```python
from build123d import *

# Parameters (mm, degrees)
SKETCH_1_W          = 10
SKETCH_1_H          = 20
SKETCH_1_R          = 1.65
EXTRUDE_1_DEPTH     = 27
FILLET_1_R          = 3
SKETCH_2_R          = 1.6
CUT_EXTRUDE_1_DEPTH = 36.057096286


with BuildPart() as part:
    # 草图1 → 凸台-拉伸1 (new body)
    with BuildSketch(Plane.XY):
        with Locations((5, -10)):
            Rectangle(SKETCH_1_W, SKETCH_1_H)
        with Locations((5, -5)):
            Circle(SKETCH_1_R, mode=Mode.SUBTRACT)
        with Locations((5, -15)):
            Circle(SKETCH_1_R, mode=Mode.SUBTRACT)
    extrude(amount=EXTRUDE_1_DEPTH)

    # 圆角1
    fillet_1_edges = [part.edges().sort_by_distance(p)[0] for p in [
        (0, 0, 13.5),
        (10, 0, 13.5),
        (10, -20, 13.5),
        (0, -20, 13.5),
    ]]
    fillet(fillet_1_edges, radius=FILLET_1_R)

    # 草图2 → 切除-拉伸1 (cut, through all)
    with BuildSketch(Plane(origin=(10, 0, 0), x_dir=(0, 0, -1), z_dir=(1, 0, 0))):
        with Locations(Location((-21, -10, 0), (0, 0, 90))):
            Circle(SKETCH_2_R)
        with Locations(Location((-6, -10, 0), (0, 0, 90))):
            Circle(SKETCH_2_R)
    extrude(amount=-CUT_EXTRUDE_1_DEPTH, mode=Mode.SUBTRACT)


solid = part.part
```
For this review, take the finished solid that the model builds, in its own axes (mm). Coordinates: 2 decimals unless noted, no trailing zeros. Loops run counter-clockwise (first coordinate to the right, second up) from the corner with the lowest first, then second, coordinate; pieces in that order, holes last.
1. Mouldability with a two-part tool opening along Y and no side actions: class faces 1 (the flat face through (0, -10, 13)), 2 (the flat face through (5, 0, 13)), 3 (the cylindrical face through (3.35, -4.93, 13.31)) as +Y half, -Y half, draft (parallel to the pull), parting line (faces both ways), or undercut.
2. Add section B-B, the plane z = 21. Give the boundary of the cut face in (x, y).
3. Insertion check: P1, Ø1, axis at x = 2, z = 12.5, coming from the -Y side; P2, Ø4, axis at x = 5, y = -15, coming from the +Z side. Each pin has a flat end and moves straight along its axis. Give the tip position at first contact, or say it passes through.
4. For line 1 (Y direction, x = 5, z = 19.25); line 2 (Y direction, x = 6.5, z = 18.5); line 3 (Y direction, x = 5, z = 7), list the stretches that pass through material, from the lowest coordinate up.
5. Add section A-A, the plane x = 5. Give the boundary of the cut face in (y, z), then the cut area to 3 significant figures.
6. Add section D-D, the plane y = -10. Give the boundary of the cut face in (x, z).
7. Add section C-C, the plane y = -15. Give the boundary of the cut face in (x, z).
Result:
1. face 1: draft
1. face 2: +Y half
1. face 3: undercut
2. outline: (0, -17) arc R3 ccw to (3, -20) - (7, -20) arc R3 ccw to (10, -17) - (10, -11.6) - (0, -11.6) - close; (0, -8.4) - (10, -8.4) - (10, -3) arc R3 ccw to (7, 0) - (3, 0) arc R3 ccw to (0, -3) - close; hole circle Ø3.3 at (5, -15); hole circle Ø3.3 at (5, -5)
3. P1: stops at y = -19.96
3. P2: stops at z = 27
4. line 1: y = -20 to -16.65, -13.35 to -6.65, -3.35 to 0
4. line 2: y = -20 to -15.69, -14.31 to -5.69, -4.31 to 0
4. line 3: y = -20 to -16.65, -13.35 to -11.25, -8.75 to -6.65, -3.35 to 0
5. outline: (-20, 0) - (-16.65, 0) - (-16.65, 27) - (-20, 27) - close; (-13.35, 0) - (-6.65, 0) - (-6.65, 27) - (-13.35, 27) - close; (-3.35, 0) - (0, 0) - (0, 27) - (-3.35, 27) - close; hole circle Ø3.2 at (-10, 6); hole circle Ø3.2 at (-10, 21)
5. area: 346 mm2
6. outline: (0, 0) - (10, 0) - (10, 4.4) - (0, 4.4) - close; (0, 7.6) - (10, 7.6) - (10, 19.4) - (0, 19.4) - close; (0, 22.6) - (10, 22.6) - (10, 27) - (0, 27) - close
7. outline: (0, 0) - (3.35, 0) - (3.35, 27) - (0, 27) - close; (6.65, 0) - (10, 0) - (10, 27) - (6.65, 27) - close
